Part model, mm, in its own coordinate system. A direction names the side the tool comes from. Give positions to 0.01 mm unless a question says otherwise; leave off trailing zeros. Order: outer loops, then holes, each group sorted by start corner. A loop starts at its lowest first (then second) coordinate and runs counter-clockwise, first axis right, second up.
1. Which spindle directions (+Z, -Z, +X, -X, +Y, -Y) get a long thin tool onto all of the face, cutting with end or side? Do faces 5 (the flat face through (-72, 0.6, -2)), 6 (the cylindrical face through (-39.706, 2.071, 10.652)), 7 (the cylindrical face through (40.93, 2.07, -11.06)). Say none if no direction does.
2. Mould opens along X. For faces 1 (the conical face through (81.79, 5.03, 0.44)), 2 (the conical face through (-77.79, 5.03, 0.36)), 3 (the cylindrical face through (-71.387, 0.296, 2.168)), 4 (the flat face through (1, 0, 0)) say: +X half, -X half, draft (parallel to the pull), parting line (faces both ways), or undercut.
3. Drop flat-ended pins along their axis: pin 1 Ø2 at (y, z) = (2.5, 10.5) entering from -X; pin 2 Ø2 at (x, y) = (-60.5, 2) entering from -Z; pin 3 Ø0.6 at (x, y) = (-60.5, 1.5) entering from +Z. Give the stop position or say it passes through.
4. Slice it at C-C on x = -8.5. List the corners of the cut face in (y, z), and give its area (3 significant figures).
5. Slice it at A-A on z = 0. List the corners of the cut face in (x, y) (3 decimals).
6. Probe line 1 (X direction, y = 2.9, z = 0) (3 decimals); line 2 (X direction, y = 2.25, z = -8) (3 decimals); line 3 (Z direction, x = -1, y = 0.35). List the from-to ranges inside material, lowest first.
7. Slice it at B-B on y = 1.55. Give the number of separate pieces and of enclosed holes in the cut face, and give its area (3 significant figures).
from build123d import *

# Parameters (mm, degrees)
SKETCH1_R           = 12.15
SKETCH1_R_2         = 16.15
BOSS_EXTRUDE1_DEPTH = 5.2
CUT_EXTRUDE1_DEPTH  = 86.410366028
FILLET1_R           = 30
CHAMFER1_SIZE       = 1
SKETCH2_R           = 14.75534968
SKETCH2_R_2         = 10
SKETCH2_R_3         = 19.025242353
SKETCH2_R_4         = 14
BOSS_EXTRUDE2_DEPTH = 0.6


with BuildPart() as part:
    # Sketch1 → Boss-Extrude1 (new body)
    with BuildSketch(Plane(origin=(0, 0, 0), x_dir=(1, 0, 0), z_dir=(0, 1, 0))):
        with BuildLine():
            Line((50.6952797, -21), (61.625, -21))
            ThreePointArc((61.625, -21), (82.625, 0), (61.625, 21))
            Line((61.625, 21), (50.6952797, 21))
            ThreePointArc((50.6952797, 21), (44.646090821, 13.026866227), (35.106613419, 10))
            Line((35.106613419, 10), (-35.106613419, 10))
            ThreePointArc((-35.106613419, 10), (-44.646090821, 13.026866227), (-50.6952797, 21))
            Line((-50.6952797, 21), (-61.625, 21))
            ThreePointArc((-61.625, 21), (-82.625, 0), (-61.625, -21))
            Line((-61.625, -21), (-50.6952797, -21))
            ThreePointArc((-50.6952797, -21), (-44.646090821, -13.026866227), (-35.106613419, -10))
            Line((-35.106613419, -10), (35.106613419, -10))
            ThreePointArc((35.106613419, -10), (44.646090821, -13.026866227), (50.6952797, -21))
        make_face()
        with Locations(Location((-61.625, 0, 0), (0, 0, 270))):
            Circle(SKETCH1_R, mode=Mode.SUBTRACT)
        with Locations(Location((61.625, 0, 0), (0, 0, 270))):
            Circle(SKETCH1_R_2, mode=Mode.SUBTRACT)
    extrude(amount=BOSS_EXTRUDE1_DEPTH)

    # Sketch4 → Cut-Extrude1 (cut, through all)
    with BuildSketch(Plane(origin=(0, 5.2, 0), x_dir=(1, 0, 0), z_dir=(0, 1, 0))):
        with BuildLine():
            Line((-61.625, 17), (-38.970543198, 17))
            Line((-38.970543198, 17), (-43.407950199, 33.342917206))
            Line((-43.407950199, 33.342917206), (-92.984497382, 23.090976894))
            Line((-92.984497382, 23.090976894), (-92.984497382, -9.501012459))
            Line((-92.984497382, -9.501012459), (-86.710921967, -27.097626428))
            Line((-86.710921967, -27.097626428), (-50.736883487, -31.973137348))
            Line((-50.736883487, -31.973137348), (-37.899444956, -29.584754809))
            Line((-37.899444956, -29.584754809), (-38.970543198, -17))
            Line((-38.970543198, -17), (-61.625, -17))
            ThreePointArc((-61.625, -17), (-78.625, 0), (-61.625, 17))
        make_face()
    extrude(amount=-CUT_EXTRUDE1_DEPTH, mode=Mode.SUBTRACT)

    # Fillet1
    # the kernel refuses this fillet: 30 mm, written as the material it takes off along each edge
    with BuildSketch(Plane(origin=(50.6952797, -27.324300751, -21), x_dir=(-0.5657553203908781, 0, 0.824573172889717), z_dir=(0, 1, 0))) as fillet1_piece_1:
        with BuildLine():
            CenterArc((16.192535549, 28.995119506), FILLET1_R, 221.766169003, 33.362358022)
            Line((-6.18354741, 9.012354147), (-6.631069069, 8.61269884))
            ThreePointArc((-6.631069069, 8.61269884), (-3.586517609, 4.166723881), (-0.494743904, -0.339453192))
            Line((-0.494743904, -0.339453192), (0.153990967, -0.57990239))
            ThreePointArc((0.153990967, -0.57990239), (4.246493598, -0.04578326), (8.338996228, -0.57990239))
            Line((8.338996228, -0.57990239), (8.492987195, 0))
        make_face()
    extrude(amount=59.848601502, mode=Mode.SUBTRACT)
    with BuildSketch(Plane(origin=(50.6952797, -27.324300751, 21), x_dir=(1, 0, 0), z_dir=(0, 1, 0))) as fillet1_piece_2:
        with BuildLine():
            CenterArc((14.747584551, 29.756073541), FILLET1_R, 229.326231532, 33.362358022)
            Line((-4.804952692, 7.003089399), (-5.196003436, 6.548029716))
            ThreePointArc((-5.196003436, 6.548029716), (-2.440227994, 3.475642576), (-0.565293163, -0.201106042))
            Line((-0.565293163, -0.201106042), (0, -0.6))
            ThreePointArc((0, -0.6), (5.46486015, -0.6), (10.853363015, -0.595121471))
            Line((10.853363015, -0.595121471), (10.9297203, 0))
        make_face()
    extrude(amount=59.848601502, mode=Mode.SUBTRACT)
    with BuildSketch(Plane(origin=(-48.621069029, 32.785704602, -17), x_dir=(-1, 0, 0), z_dir=(0, -1, 0))) as fillet1_piece_3:
        with BuildLine():
            CenterArc((11.034281841, -30), FILLET1_R, 90, 31.830687787)
            Line((-4.788045906, -4.511690039), (-5.104492461, -4.00192384))
            ThreePointArc((-5.104492461, -4.00192384), (-2.578998673, -2.059538928), (-0.490075881, 0.34615839))
            Line((-0.490075881, 0.34615839), (0, 0.6))
            Line((0, 0.6), (11.034281841, 0.6))
            Line((11.034281841, 0.6), (11.034281841, 0))
        make_face()
    extrude(amount=60.371409204, mode=Mode.SUBTRACT)
    with BuildSketch(Plane(origin=(-48.621069029, 32.785704602, 17), x_dir=(0.7277982616759969, 0, -0.6857912877117915), z_dir=(0, -1, 0))) as fillet1_piece_4:
        with BuildLine():
            CenterArc((12.543007489, -29.401162203), FILLET1_R, 101.467181472, 31.830687787)
            Line((-8.030731143, -7.567214353), (-8.442205915, -7.130535396))
            Line((-8.442205915, -7.130535396), (-0.411474773, 0.436678957))
            Line((-0.411474773, 0.436678957), (0.119283966, 0.588023244))
            ThreePointArc((0.119283966, 0.588023244), (3.289404605, 0.269725969), (6.459525243, 0.588023244))
            Line((6.459525243, 0.588023244), (6.578809209, 0))
        make_face()
    extrude(amount=60.371409204, mode=Mode.SUBTRACT)

    # Chamfer1
    # the kernel refuses this chamfer: 1 mm, written as the material it takes off along each edge
    with BuildSketch(Plane(origin=(61.625, 5.2, 0), x_dir=(-0.12235070165055927, 0, 0.9924869297908239), z_dir=(-0.9924869297908239, 0, -0.12235070165055927))) as chamfer1_piece_1:
        Polygon((21 - CHAMFER1_SIZE, 0), (21, -CHAMFER1_SIZE), (21, 0), align=None)
    revolve(axis=Axis((61.625, 5.2, 0), (0, 1, 0)), revolution_arc=194.055575488, mode=Mode.SUBTRACT)
    with BuildSketch(Plane(origin=(35.106613419, 5.2, -26.545750746), x_dir=(0.6517512414299695, 0, 0.7584328047325575), z_dir=(0.7584328047325575, 0, -0.6517512414299695))) as chamfer1_piece_2:
        Polygon((16.545750746 + CHAMFER1_SIZE, 0), (16.545750746, CHAMFER1_SIZE), (16.545750746, 0), align=None)
    revolve(axis=Axis((35.106613419, 5.2, -26.545750746), (0, -1, 0)), revolution_arc=40.673768468, mode=Mode.SUBTRACT)
    with BuildSketch(Plane(origin=(35.106613419, 5.2, -10), x_dir=(0, 0, 1), z_dir=(-1, 0, 0))) as chamfer1_piece_3:
        Polygon((CHAMFER1_SIZE, 0), (0, -CHAMFER1_SIZE), (0, 0), align=None)
    extrude(amount=70.213226838, mode=Mode.SUBTRACT)
    with BuildSketch(Plane(origin=(-61.625, 5.2, 0), x_dir=(0, 0, 1), z_dir=(1, 0, 0))) as chamfer1_piece_4:
        Polygon((17 - CHAMFER1_SIZE, 0), (17, CHAMFER1_SIZE), (17, 0), align=None)
    revolve(axis=Axis((-61.625, 5.2, 0), (0, -1, 0)), revolution_arc=180, mode=Mode.SUBTRACT)
    with BuildSketch(Plane(origin=(-61.625, 5.2, -17), x_dir=(0, 0, 1), z_dir=(1, 0, 0)), Plane(origin=(-59.65535087, 5.2, 17), x_dir=(0, 0, -1), z_dir=(-1, 0, 0))) as chamfer1_piece_5:
        Polygon((CHAMFER1_SIZE, 0), (0, CHAMFER1_SIZE), (0, 0), align=None)
    extrude(amount=1.96964913, mode=Mode.SUBTRACT)
    with BuildSketch(Plane(origin=(-35.106613419, 5.2, 26.545750746), x_dir=(-0.5274109249013418, 0, -0.8496103320315208), z_dir=(-0.8496103320315208, 0, 0.5274109249013418))) as chamfer1_piece_6:
        Polygon((16.545750746, CHAMFER1_SIZE), (16.545750746 + CHAMFER1_SIZE, 0), (16.545750746, 0), align=None)
    revolve(axis=Axis((-35.106613419, 5.2, 26.545750746), (0, -1, 0)), revolution_arc=31.830687787, mode=Mode.SUBTRACT)
    with BuildSketch(Plane(origin=(-35.106613419, 5.2, 10), x_dir=(0, -1, 0), z_dir=(1, 0, 0))) as chamfer1_piece_7:
        Polygon((CHAMFER1_SIZE, 0), (0, CHAMFER1_SIZE), (0, 0), align=None)
    extrude(amount=70.213226838, mode=Mode.SUBTRACT)
    with BuildSketch(Plane(origin=(-61.625, 5.2, 0), x_dir=(0, 0, 1), z_dir=(-1, 0, 0))) as chamfer1_piece_8:
        Polygon((12.15 + CHAMFER1_SIZE, 0), (12.15, -CHAMFER1_SIZE), (12.15, 0), align=None)
    revolve(axis=Axis((-61.625, 5.2, 0), (0, 1, 0)), mode=Mode.SUBTRACT)
    with BuildSketch(Plane(origin=(61.625, 5.2, 0), x_dir=(0, 0, 1), z_dir=(-1, 0, 0))) as chamfer1_piece_9:
        Polygon((16.15 + CHAMFER1_SIZE, 0), (16.15, -CHAMFER1_SIZE), (16.15, 0), align=None)
    revolve(axis=Axis((61.625, 5.2, 0), (0, 1, 0)), mode=Mode.SUBTRACT)
    with BuildSketch(Plane(origin=(-35.106613419, 5.2, -26.545750746), x_dir=(0, 0, 1), z_dir=(1, 0, 0))) as chamfer1_piece_10:
        Polygon((16.545750746 + CHAMFER1_SIZE, 0), (16.545750746, CHAMFER1_SIZE), (16.545750746, 0), align=None)
    revolve(axis=Axis((-35.106613419, 5.2, -26.545750746), (0, -1, 0)), revolution_arc=31.830687787, mode=Mode.SUBTRACT)
    with BuildSketch(Plane(origin=(35.106613419, 5.2, 26.545750746), x_dir=(0, 0, -1), z_dir=(-1, 0, 0))) as chamfer1_piece_11:
        Polygon((16.545750746 + CHAMFER1_SIZE, 0), (16.545750746, CHAMFER1_SIZE), (16.545750746, 0), align=None)
    revolve(axis=Axis((35.106613419, 5.2, 26.545750746), (0, -1, 0)), revolution_arc=40.673768468, mode=Mode.SUBTRACT)
    with BuildSketch(Plane(origin=(65.442864251, 5.2, -8.756073541), x_dir=(0.1292120287500912, 0, 0.9916169883711581), z_dir=(0.9916169883711581, 0, -0.1292120287500912))) as chamfer1_piece_12:
        Polygon((30 - CHAMFER1_SIZE, 0), (30, CHAMFER1_SIZE), (30, 0), align=None)
    revolve(axis=Axis((65.442864251, 5.2, -8.756073541), (0, -1, 0)), revolution_arc=48.097829324, mode=Mode.SUBTRACT)
    with BuildSketch(Plane(origin=(65.442864251, 5.2, 8.756073541), x_dir=(-0.6517512414300072, 0, -0.7584328047325251), z_dir=(-0.7584328047325251, 0, 0.6517512414300072))) as chamfer1_piece_13:
        Polygon((30 - CHAMFER1_SIZE, 0), (30, CHAMFER1_SIZE), (30, 0), align=None)
    revolve(axis=Axis((65.442864251, 5.2, 8.756073541), (0, -1, 0)), revolution_arc=48.097829324, mode=Mode.SUBTRACT)
    with BuildSketch(Plane(origin=(-59.65535087, 5.2, -13), x_dir=(0, 0, 1), z_dir=(-1, 0, 0))) as chamfer1_piece_14:
        Polygon((30 - CHAMFER1_SIZE, 0), (30, -CHAMFER1_SIZE), (30, 0), align=None)
    revolve(axis=Axis((-59.65535087, 5.2, -13), (0, 1, 0)), revolution_arc=31.830687787, mode=Mode.SUBTRACT)
    with BuildSketch(Plane(origin=(-59.65535087, 5.2, 13), x_dir=(0.5274109249013516, 0, -0.8496103320315149), z_dir=(0.8496103320315149, 0, 0.5274109249013516))) as chamfer1_piece_15:
        Polygon((30 - CHAMFER1_SIZE, 0), (30, -CHAMFER1_SIZE), (30, 0), align=None)
    revolve(axis=Axis((-59.65535087, 5.2, 13), (0, 1, 0)), revolution_arc=31.830687787, mode=Mode.SUBTRACT)

    # Sketch2 → Boss-Extrude2 (add)
    # profile 1 of 2: a face of its own
    with BuildSketch(Plane.XZ):
        with Locations((-61.625, 0)):
            Circle(SKETCH2_R)
        with Locations(Location((-61.625, 0, 0), (0, 0, 270))):
            Circle(SKETCH2_R_2, mode=Mode.SUBTRACT)
    # profile 2 of 2: a face of its own
    with BuildSketch(Plane.XZ):
        with Locations((61.625, 0)):
            Circle(SKETCH2_R_3)
        with Locations(Location((61.625, 0, 0), (0, 0, 270))):
            Circle(SKETCH2_R_4, mode=Mode.SUBTRACT)
    extrude(amount=-BOSS_EXTRUDE2_DEPTH)


solid = part.part
Data:
1. face 5: +Y
1. face 6: +Z, +Y, -Y
1. face 7: -Z, +Y, -Y
2. face 1: +X half
2. face 2: -X half
2. face 3: undercut
2. face 4: draft
3. pin 1: stops at x = -75.72
3. pin 2: stops at z = -17
3. pin 3: stops at z = 17
4. outline: (0, -10) - (4.2, -10) - (5.2, -9) - (5.2, 9) - (4.2, 10) - (0, 10) - close
4. area: 103 mm2
5. outline: (-78.625, 0) - (-71.625, 0) - (-71.625, 0.6) - (-73.775, 0.6) - (-73.775, 4.2) - (-74.775, 5.2) - (-77.625, 5.2) - (-78.625, 4.2) - close; (-51.625, 0) - (47.625, 0) - (47.625, 0.6) - (45.475, 0.6) - (45.475, 4.2) - (44.475, 5.2) - (-48.475, 5.2) - (-49.475, 4.2) - (-49.475, 0.6) - (-51.625, 0.6) - close; (75.625, 0) - (82.625, 0) - (82.625, 4.2) - (81.625, 5.2) - (78.775, 5.2) - (77.775, 4.2) - (77.775, 0.6) - (75.625, 0.6) - close
6. line 1: x = -78.625 to -73.775, -49.475 to 45.475, 77.775 to 82.625
6. line 2: x = -76.625 to -70.77, -52.48 to 47.596, 75.654 to 81.041
6. line 3: z = -10 to 10
7. separate pieces: 1
7. enclosed holes: 2
7. area: 2,840 mm2
